Job drawing, mm, ordinate dimensions from the low corner. One solid piece. A direction names the side the tool comes from. Coordinates: 2 decimals unless noted, no trailing zeros. Order: outer loops, then holes, each group sorted by start corner. A loop starts at its lowest first (then second) coordinate and runs counter-clockwise, first axis right, second up. Notation, with made-up numbers: (48, 49) - (93, 49) arc R16 cw to (93, 68) - close; hole circle Ø1 at (-2, 56.25). An arc over 180 degrees is marked (long way). Return JSON: item names as keys, results as strings.
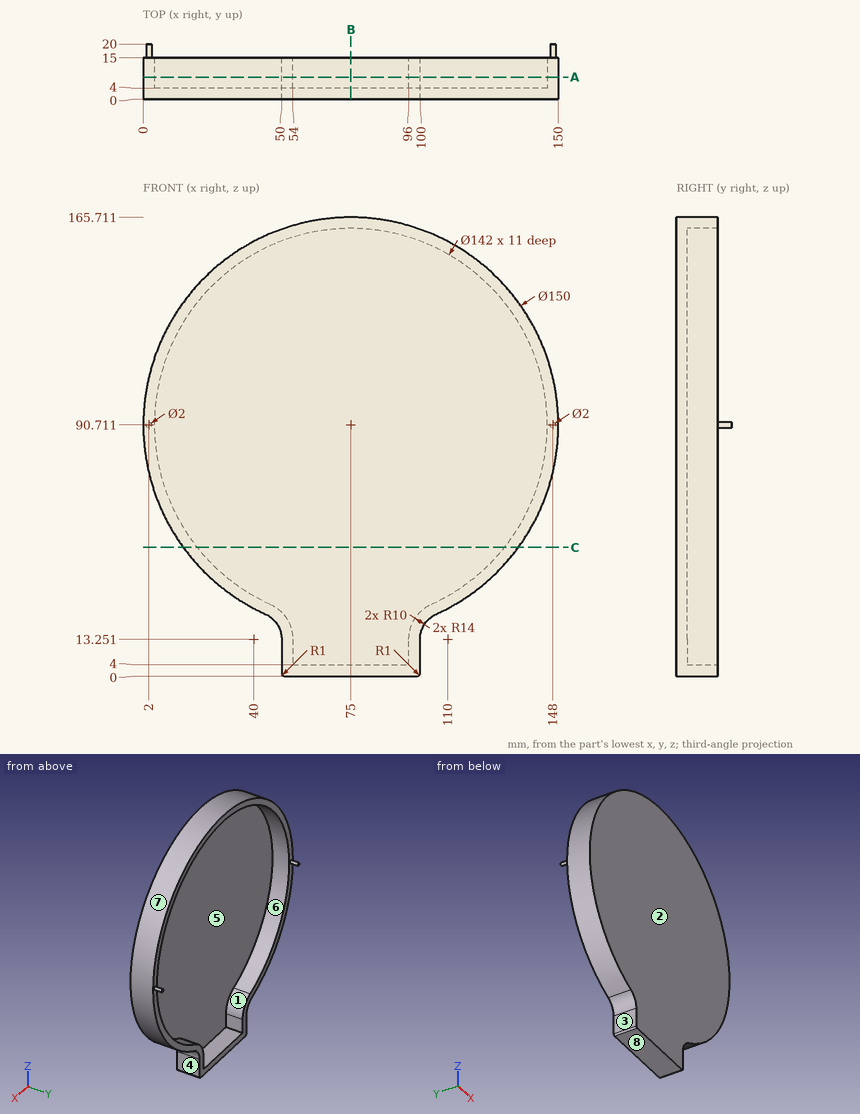
1. Mould opens along Z. For the marked faces 5, 6, 7 and 8 say: pulls with the +Z half, pulls with the -Z half, needs draft (parallel to the pull), parting line crosses it, or undercut.
Check values:
{"face 5": "undercut", "face 6": "undercut", "face 7": "parting line crosses it", "face 8": "pulls with the -Z half"}
2. Probe L1, parallel to X at y = 5.75, z = 116; L2, parallel to Y at x = 105.5, z = 54.5; L3, parallel to X at y = 5.25, z = 151. List the from-to ranges inside material, lowest first.
Check values:
{"L1": "4.39 to 8.66, 141.34 to 145.61", "L2": "0 to 4", "L3": "30.39 to 37.5, 112.5 to 119.61"}
3. Cut at C-C on z = 46.5. Give the cut face in (x, y) (1 decimal), plus the area to 3 significant figures.
Check values:
{"outline": "(14.4, 0) - (135.6, 0) - (135.6, 15) - (130.6, 15) - (130.6, 4) - (19.4, 4) - (19.4, 15) - (14.4, 15) - close", "area": "595 mm²"}
4. Drop flat-ended pins along their axis: pin 1 (5 mm diameter, centred on x = 17, y = 9.5, fed in from -Z) (1 decimal); pin 2 (8 mm diameter, centred on x = 112, y = 9, fed in from -Z); pin 3 (10 mm diameter, centred on y = 10.5, z = 115, fed in from +X). Give the stop position or say it passes through.
Check values:
{"pin 1": "z = 40.3", "pin 2": "z = 23.36", "pin 3": "x = 147.48"}
5. Cut at A-A on y = 8. Give the cut face in (x, z) (1 decimal).
Check values:
{"outline": "(44.1, 22.4) arc R10 cw to (50, 13.3) - (50, 1) arc R1 ccw to (51, 0) - (99, 0) arc R1 ccw to (100, 1) - (100, 13.3) arc R10 cw to (105.9, 22.4) arc R75 ccw (long way) to start; hole (45.8, 26) arc R14 cw to (54, 13.3) - (54, 4) - (96, 4) - (96, 13.3) arc R14 cw to (104.2, 26) arc R71 ccw (long way) to start"}
6. Cut at B-B on x = 75. Give the cut face in (y, z), plus the area to 3 significant figures.
Check values:
{"outline": "(0, 0) - (15, 0) - (15, 4) - (4, 4) - (4, 161.71) - (15, 161.71) - (15, 165.71) - (0, 165.71) - close", "area": "751 mm²"}
7. Tool access for the marked faces 1, 2, 3 and 4: list every direction of +Z, -Z, +X, -X, +Y, -Y with a clear straight run to the whole face (end or side of a thin tool).
Check values:
{"face 1": "+Y", "face 2": "+Z, -Z, +X, -X, -Y", "face 3": "-Z, -X, +Y, -Y", "face 4": "-Z, +X, +Y, -Y"}
